Check sheet for the modelled part. Datum: model origin and axes. Units: mm. A direction names the side the tool comes from. Round coordinates to 2 decimals unless told otherwise and drop trailing zeros. Write each loop counter-clockwise with the first axis right and the second up, starting at its lowest first coordinate (ties: lowest second). Pieces come first, ordered by that corner, then holes. Notation, with made-up numbers: M 14,-25 L 45,-25 A17 cw 45,-13 Z; hole C -31,48.5 d5. An arc over 180 degrees is marked long. Answer in a Markdown table with one row per item.
```python
from build123d import *

# Parameters (mm, degrees)
SKETCH_1_R          = 4.5
EXTRUDE_1_DEPTH     = 2
SKETCH_2_R          = 2
EXTRUDE_2_DEPTH     = 10
FILLET_1_R          = 1
CHAMFER_1_SIZE      = 0.5
CUT_EXTRUDE_1_DEPTH = 1


with BuildPart() as part:
    # 草图1 → 凸台-拉伸1 (new body)
    with BuildSketch(Plane.XY):
        Circle(SKETCH_1_R)
    extrude(amount=EXTRUDE_1_DEPTH)

    # 草图2 → 凸台-拉伸2 (add)
    with BuildSketch(Plane.XY.offset(2)):
        Circle(SKETCH_2_R)
    extrude(amount=EXTRUDE_2_DEPTH)

    # 圆角1
    fillet_1_edges = [part.edges().sort_by_distance(p)[0] for p in [
        (-4.5, 0, 0),
    ]]
    fillet(fillet_1_edges, radius=FILLET_1_R)

    # 倒角1
    chamfer_1_edges = [part.edges().sort_by_distance(p)[0] for p in [
        (-4.5, 0, 2),
    ]]
    chamfer(chamfer_1_edges, length=CHAMFER_1_SIZE)

    # 草图3 → 切除-拉伸1 (cut)
    with BuildSketch(Plane(origin=(0, 0, 0), x_dir=(-1, 0, 0), z_dir=(0, 0, -1))):
        Polygon((-0.866025404, 1.5), (-1.732050808, 0), (-0.866025404, -1.5), (0.866025404, -1.5), (1.732050808, 0), (0.866025404, 1.5), align=None)
    extrude(amount=-CUT_EXTRUDE_1_DEPTH, mode=Mode.SUBTRACT)


solid = part.part
```
1. Section check A-A, the plane x = 0. Record the cut outline in (y, z), and give its area (3 significant figures).
Found:
| item | result |
|---|---|
| outline | M -4.5,1 A1 ccw -3.5,0 L -1.5,0 L -1.5,1 L 1.5,1 L 1.5,0 L 3.5,0 A1 ccw 4.5,1 L 4.5,1.5 L 4,2 L 2,2 L 2,12 L -2,12 L -2,2 L -4,2 L -4.5,1.5 Z |
| area | 54.3 mm2 |
2. Access from +Z, -Z, +X, -X, +Y, -Y to the whole of each face (thin tool, end or side, straight path). Record for faces 4 (the face through (1.293, 0.76, 0.493)), 5 (the face through (0, 0, 12)), 6 (the face through (0, -2, 7)).
Found:
| item | result |
|---|---|
| face 4 | -Z |
| face 5 | +Z, +X, -X, +Y, -Y |
| face 6 | +Z |
3. Scan lines: L1, parallel to Y at x = 0, z = 7.5; L2, parallel to Z at x = 0.75, y = 2.75; L3, parallel to Y at x = -0.25, z = 0.5. Record each from-to range of solid material in increasing order.
Found:
| item | result |
|---|---|
| L1 | y = -2 to 2 |
| L2 | z = 0 to 2 |
| L3 | y = -4.36 to -1.5, 1.5 to 4.36 |
4. Go/stop test with flat-tipped pins: pin 1 (1.5 mm diameter, centred on x = 3, y = 2.5, fed in from -Z); pin 2 (2 mm diameter, centred on y = -2, z = 4, fed in from +X); pin 3 (4 mm diameter, centred on y = 3.5, z = 5, fed in from +X); pin 4 (0.5 mm diameter, centred on x = 0.5, z = 0.5, fed in from +Y). Record where each tip stops, or that it passes through.
Found:
| item | result |
|---|---|
| pin 1 | stops at z = 0 |
| pin 2 | stops at x = 1.73 |
| pin 3 | stops at x = 1.32 |
| pin 4 | stops at y = 4.44 |
5. Section check B-B, the plane z = 7.25. Record the cut outline in (x, y).
Found:
| item | result |
|---|---|
| outline | C 0,0 d4 |
6. Draft check along X on faces 1 (the face through (-0.59, 4.46, 1.25)), 2 (the face through (-1.305, 0.74, 0.493)), 3 (the face through (-2, -1, 2)). Enter one of: +X half, -X half, draft (parallel to the pull), parting line (faces both ways), or undercut.
Found:
| item | result |
|---|---|
| face 1 | parting line |
| face 2 | undercut |
| face 3 | draft |
